Input: dimensioned drawing with shaded views. Units: mm. Origin: part minimum x, y, z. Give positions to 0.01 mm unless a question says otherwise; leave off trailing zeros. Loops run counter-clockwise (first coordinate to the right, second up) from the corner with the lowest first, then second, coordinate; pieces in that order, holes last.
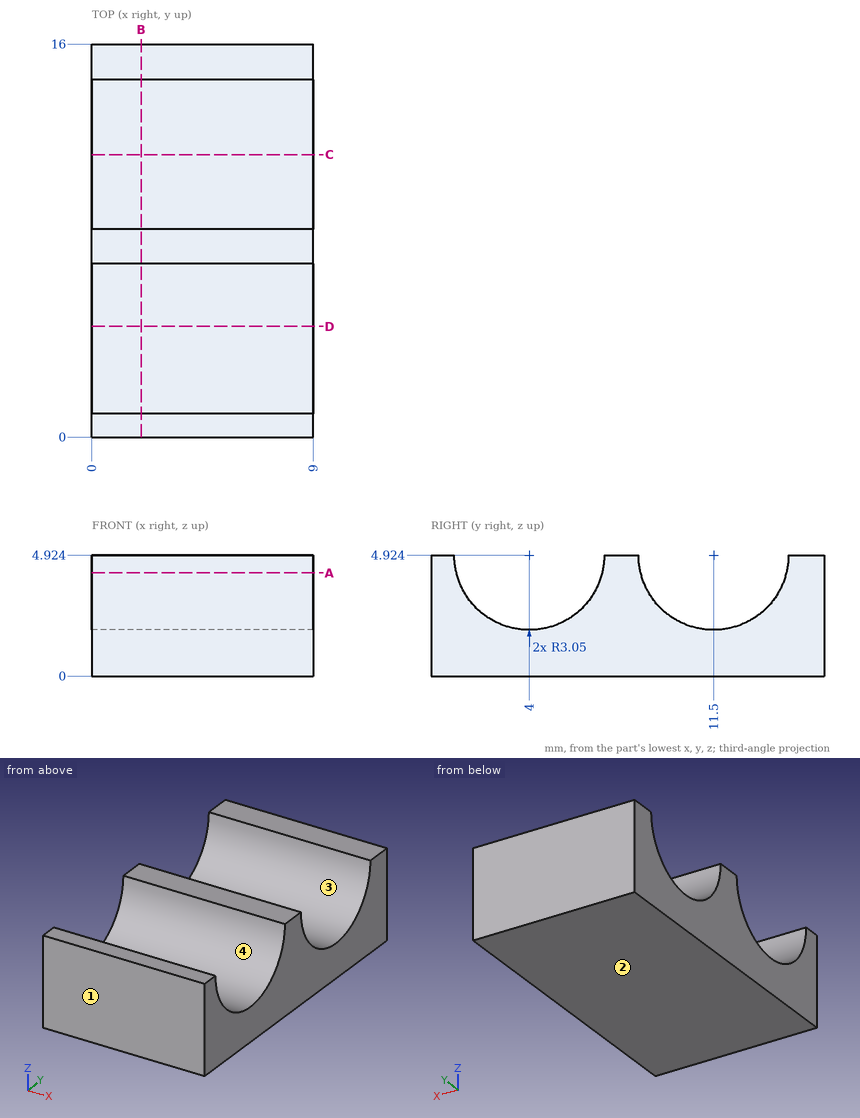
Item 1: Ray query, probe 1 along Y at (x, z) = (7.75, 3); probe 2 along Y at (x, z) = (2.5, 4.5); probe 3 along Z at (x, y) = (8.5, 6.5). Return the intervals inside material, ascending.
Values follow:
probe 1: y = 0 to 1.63, 6.37 to 9.13, 13.87 to 16
probe 2: y = 0 to 0.98, 7.02 to 8.48, 14.52 to 16
probe 3: z = 0 to 3.18
Item 2: Section query B-B on x = 2. Return loops of the section in (y, z), plus the area to 3 significant figures.
Values follow:
outline: (0, 0) - (16, 0) - (16, 4.92) - (14.55, 4.92) arc R3.05 cw to (8.45, 4.92) - (7.05, 4.92) arc R3.05 cw to (0.95, 4.92) - (0, 4.92) - close
area: 49.6 mm2
Item 3: Section query C-C on y = 11.5. Return loops of the section in (x, z), plus the area to 3 significant figures.
Values follow:
outline: (0, 0) - (9, 0) - (9, 1.87) - (0, 1.87) - close
area: 16.9 mm2
Item 4: Section query A-A on z = 4.2. Return loops of the section in (x, y).
Values follow:
outline: (0, 0) - (9, 0) - (9, 1.04) - (0, 1.04) - close; (0, 6.96) - (9, 6.96) - (9, 8.54) - (0, 8.54) - close; (0, 14.46) - (9, 14.46) - (9, 16) - (0, 16) - close
Item 5: Draft query along Y for the marked faces 1, 2, 3 and 4. Return one class per face: +Y half, -Y half, draft (parallel to the pull), parting line (faces both ways), or undercut.
Values follow:
face 1: -Y half
face 2: draft
face 3: undercut
face 4: undercut
Item 6: Section query D-D on y = 4.5. Return loops of the section in (x, z), plus the area to 3 significant figures.
Values follow:
outline: (0, 0) - (9, 0) - (9, 1.92) - (0, 1.92) - close
area: 17.2 mm2
